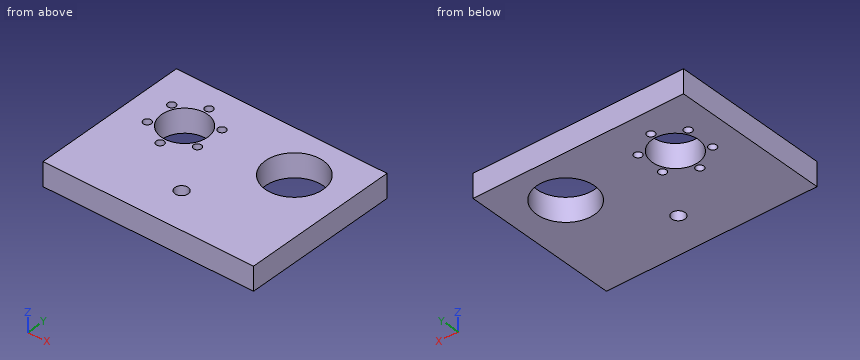
```python
from build123d import *

# Parameters (mm, degrees)
ESQUISSE1_W             = 80
ESQUISSE1_H             = 60
BOSS_EXTRU_1_DEPTH      = 9
ESQUISSE2_R             = 11
ESQUISSE2_R_2           = 8.75
ESQUISSE2_R_3           = 1.5
ENL_V_MAT_EXTRU_1_DEPTH = 101.40418318
ESQUISSE3_R             = 2.5
ENL_V_MAT_EXTRU_2_DEPTH = 101.40418318


with BuildPart() as part:
    # Esquisse1 → Boss.-Extru.1 (new body)
    with BuildSketch(Plane.XY):
        with Locations((40, 30)):
            Rectangle(ESQUISSE1_W, ESQUISSE1_H)
    extrude(amount=BOSS_EXTRU_1_DEPTH)

    # Esquisse2 → Enlèv. mat.-Extru.1 (cut, through all)
    with BuildSketch(Plane.XY.offset(9)):
        with Locations((60, 42)):
            Circle(ESQUISSE2_R)
        with Locations((20, 40)):
            Circle(ESQUISSE2_R_2)
        with Locations((20, 51)):
            Circle(ESQUISSE2_R_3)
        with Locations((29.526279442, 45.5)):
            Circle(ESQUISSE2_R_3)
        with Locations((29.526279442, 34.5)):
            Circle(ESQUISSE2_R_3)
        with Locations((20, 29)):
            Circle(ESQUISSE2_R_3)
        with Locations((10.473720558, 34.5)):
            Circle(ESQUISSE2_R_3)
        with Locations((10.473720558, 45.5)):
            Circle(ESQUISSE2_R_3)
    extrude(amount=-ENL_V_MAT_EXTRU_1_DEPTH, mode=Mode.SUBTRACT)

    # Esquisse3 → Enlèv. mat.-Extru.2 (cut, through all)
    with BuildSketch(Plane.XY.offset(9)):
        with Locations((40, 15)):
            Circle(ESQUISSE3_R)
    extrude(amount=-ENL_V_MAT_EXTRU_2_DEPTH, mode=Mode.SUBTRACT)


solid = part.part
```
Check sheet for the modelled part. Datum: model origin and axes. Units: mm. Give positions to 0.01 mm unless a question says otherwise; leave off trailing zeros. Order: outer loops, then holes, each group sorted by start corner. A loop starts at its lowest first (then second) coordinate and runs counter-clockwise, first axis right, second up. Notation, with made-up numbers: M -18.75,52.25 L 35.25,52.25 A29 ccw 35.25,88.25 Z; hole C -22,61 d3. An arc over 180 degrees is marked long. Answer in a Markdown table with one row per item.
1) Cross-section at A-A, the plane x = 38.5. Enter the section's corners in (y, z).
Filled sheet:
| item | result |
|---|---|
| outline | M 0,0 L 13,0 L 13,9 L 0,9 Z; M 17,0 L 60,0 L 60,9 L 17,9 Z |
2) Gauge pin test, flat end, axial feed: P1, Ø16, axis at x = 20, y = 40, coming from the -Z side. Record the tip position at first contact, or that the pin passes through.
Filled sheet:
| item | result |
|---|---|
| P1 | passes through |
3) Cross-section at D-D, the plane x = 20. Enter the section's corners in (y, z), plus the area to 4 significant figures.
Filled sheet:
| item | result |
|---|---|
| outline | M 0,0 L 27.5,0 L 27.5,9 L 0,9 Z; M 30.5,0 L 31.25,0 L 31.25,9 L 30.5,9 Z; M 48.75,0 L 49.5,0 L 49.5,9 L 48.75,9 Z; M 52.5,0 L 60,0 L 60,9 L 52.5,9 Z |
| area | 328.5 mm2 |
4) Cross-section at C-C, the plane y = 29. Enter the section's corners in (x, z).
Filled sheet:
| item | result |
|---|---|
| outline | M 0,0 L 18.5,0 L 18.5,9 L 0,9 Z; M 21.5,0 L 80,0 L 80,9 L 21.5,9 Z |
5) Thickness scan on L1, parallel to X at y = 50, z = 2; L2, parallel to X at y = 32, z = 7.5; L3, parallel to Y at x = 41, z = 6.25. Record the ranges inside material, lowest first. Write a range as [from, to].
Filled sheet:
| item | result |
|---|---|
| L1 | x = [0, 18.88], [21.12, 52.45], [67.55, 80] |
| L2 | x = [0, 16.46], [23.54, 55.42], [64.58, 80] |
| L3 | y = [0, 12.71], [17.29, 60] |
6) Cross-section at B-B, the plane z = 7. Count the separate pieces of the cut face and the enclosed holes in it, plus the area to 3 significant figures.
Filled sheet:
| item | result |
|---|---|
| separate pieces | 1 |
| enclosed holes | 9 |
| area | 4,120 mm2 |
